CAD build for the part. Positions are in the model's coordinates, mm. Face numbers are marked on the shaded views. A direction names the side the tool comes from. Coordinates: 2 decimals unless noted, no trailing zeros. Loops run counter-clockwise (first coordinate to the right, second up) from the corner with the lowest first, then second, coordinate; pieces in that order, holes last. Notation, with made-up numbers: (63.5, 65) -> (119.5, 65) arc R21 ccw to (119.5, 95) -> close; hole circle Ø10 at (12.25, 85). An arc over 180 degrees is marked (long way). Return JSON: item names as keys, results as strings. Group by question number.
(1) Saw through at B-B on y = 0.5. Write the cut outline in (x, z), then the cut area to 3 significant figures.
(2) Saw through at C-C on z = 0.65. Write the cut outline in (x, y), then the cut area to 3 significant figures.
(3) Probe L1, parallel to X at y = 12.5, z = 0.95; L2, parallel to X at y = 1.75, z = 4.3; L3, parallel to X at y = 8, z = 1.5. List the from-to ranges inside material, lowest first.
(4) Tool access for the marked faces 4, 5, 6 and 7: list every direction of +Z, -Z, +X, -X, +Y, -Y with a clear straight run to the whole face (end or side of a thin tool).
(5) Flat gauge pins, fed straight in: pin 1 Ø1.6 at (y, z) = (1.16, 2.25) entering from -X; pin 2 Ø2 at (y, z) = (2.5, 3) entering from +X; pin 3 Ø2 at (y, z) = (2, 1) entering from -X. Where does each tip first touch, or does it go through?
(6) Saw through at D-D on x = 8. Write the cut outline in (y, z), then the cut area to 3 significant figures.
(7) Saw through at A-A on z = 2.75. Write the cut outline in (x, y).
(8) Mould opens along X. For the marked faces 1, 2 and 3 say: pulls with the +X half, pulls with the -X half, needs draft (parallel to the pull), parting line crosses it, or undercut.
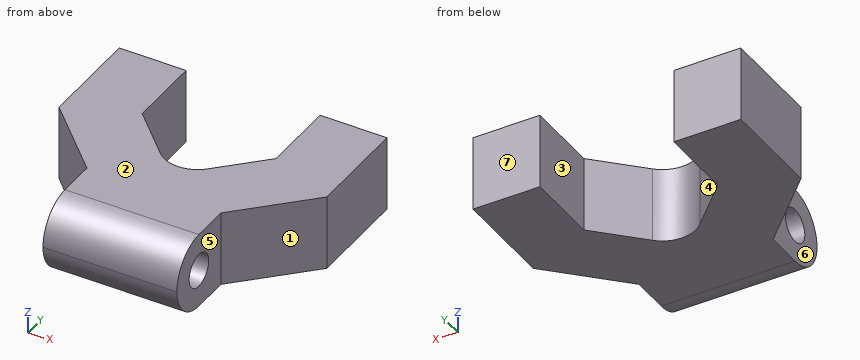
```python
from build123d import *

# Parameters (mm, degrees)
F1_DEPTH = 4.5
F2_R     = 2
F4_R     = 1
F5_DEPTH = 25
F6_R     = 2.25
F7_R     = 2.24999


# Not quite as in the source:
# - a fillet or chamfer is up to 0.001 mm smaller than in the source, because OpenCascade refuses the exact size


with BuildPart() as f1:
    # F0 (on Top) → F1 (new body)
    with BuildSketch(Plane.XY):
        Polygon((12.6486692298, 5.0720985499), (12.6486692298, -1.0879014501), (16.6486692298, -1.0879014501), (16.6486692298, 3.4120985499), (20.6486692298, 7.4120985499), (20.6486692298, 13.5720985499), (16.6486692298, 13.5720985499), (16.6486692298, 9.0720985499), align=None)
        Polygon((8.6486692298, -1.0879014501), (12.6486692298, -1.0879014501), (12.6486692298, 5.0720985499), (8.6486692298, 9.0720985499), (8.6486692298, 13.5720985499), (4.6486692298, 13.5720985499), (4.6486692298, 7.4120985499), (8.6486692298, 3.4120985499), align=None)
    extrude(amount=F1_DEPTH)

    # F2
    f2_edges = [f1.edges().sort_by_distance(p)[0] for p in [
        (12.648669, 5.072099, 2.25),
    ]]
    fillet(f2_edges, radius=F2_R)

    # F4 (on face) → F5 (cut)
    with BuildSketch(Plane.YZ.offset(16.6486692298)):
        with Locations((1.1620985499, 2.25)):
            Circle(F4_R)
    extrude(amount=-F5_DEPTH, mode=Mode.SUBTRACT)

    # F6
    f6_edges = [f1.edges().sort_by_distance(p)[0] for p in [
        (12.648669, -1.087901, 0),
    ]]
    fillet(f6_edges, radius=F6_R)

    # F7 (radius 2.25 in the source; OpenCascade refuses exactly that, so slightly less here)
    f7_edges = [f1.edges().sort_by_distance(p)[0] for p in [
        (12.648669, -1.087901, 4.5),
    ]]
    fillet(f7_edges, radius=F7_R)


solid = f1.part
```
Geometry results:
{
 "1": {"outline": "(8.65, 0.1) -> (16.65, 0.1) -> (16.65, 1.5) -> (8.65, 1.5) -> close; (8.65, 3) -> (16.65, 3) -> (16.65, 4.4) -> (8.65, 4.4) -> close", "area": "22.4 mm²"},
 "2": {"outline": "(4.65, 7.41) -> (8.65, 3.41) -> (8.65, -0.42) -> (16.65, -0.42) -> (16.65, 3.41) -> (20.65, 7.41) -> (20.65, 13.57) -> (16.65, 13.57) -> (16.65, 9.07) -> (14.06, 6.49) arc R2 cw to (11.23, 6.49) -> (8.65, 9.07) -> (8.65, 13.57) -> (4.65, 13.57) -> close", "area": "126 mm²"},
 "3": {"L1": "4.65 to 8.65, 16.65 to 20.65", "L2": "8.65 to 16.65", "L3": "4.65 to 9.72, 15.58 to 20.65"},
 "4": {"face 4": "+Z, -Z, +Y", "face 5": "+Z, -Z, +X, -Y", "face 6": "+Z, -Z, -X, -Y", "face 7": "+Z, -Z, +X, -X, +Y"},
 "5": {"pin 1": "through", "pin 2": "x = 16.74", "pin 3": "x = 8.65"},
 "6": {"outline": "(4.06, 0) -> (13.57, 0) -> (13.57, 4.5) -> (4.06, 4.5) -> close", "area": "42.8 mm²"},
 "7": {"outline": "(4.65, 7.41) -> (8.65, 3.41) -> (8.65, 2.03) -> (16.65, 2.03) -> (16.65, 3.41) -> (20.65, 7.41) -> (20.65, 13.57) -> (16.65, 13.57) -> (16.65, 9.07) -> (14.06, 6.49) arc R2 cw to (11.23, 6.49) -> (8.65, 9.07) -> (8.65, 13.57) -> (4.65, 13.57) -> close; (8.65, -1.03) -> (16.65, -1.03) -> (16.65, 0.3) -> (8.65, 0.3) -> close"},
 "8": {"face 1": "pulls with the +X half", "face 2": "needs draft", "face 3": "undercut"}
}
